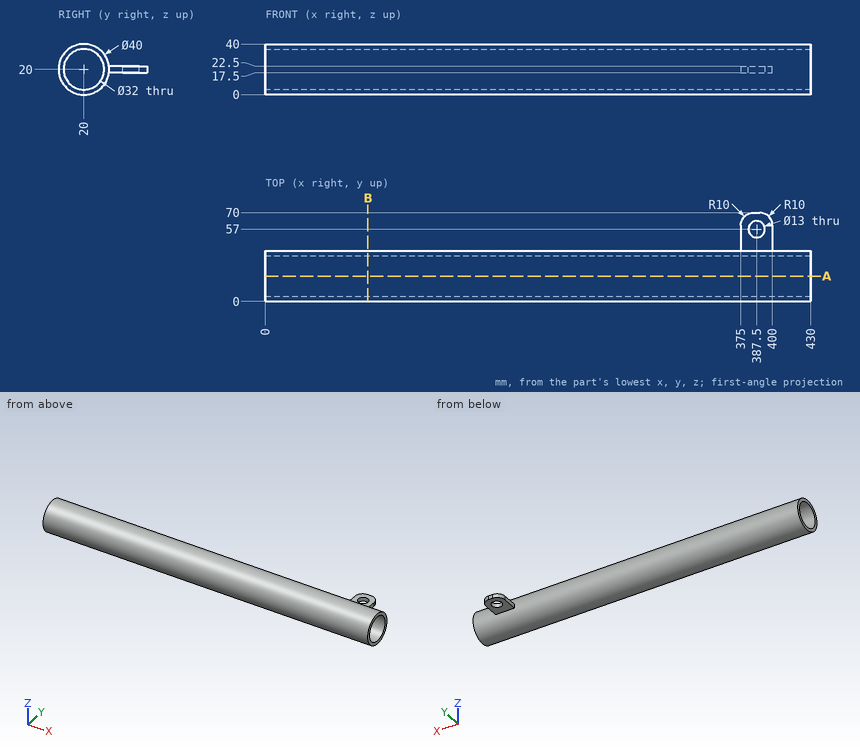
Input: dimensioned drawing with shaded views. Units: mm. Origin: part minimum x, y, z. Give positions to 0.01 mm unless a question says otherwise; leave off trailing zeros. Order: outer loops, then holes, each group sorted by start corner. A loop starts at its lowest first (then second) coordinate and runs counter-clockwise, first axis right, second up. Notation, with made-up numbers: (65.25, 35) -> (108.25, 35) arc R36 ccw to (108.25, 71) -> close; hole circle Ø7 at (87, -18). An arc over 180 degrees is marked (long way). Use a Markdown table: item, result.
1) Section query B-B, the plane x = 81. Return the cut outline in (y, z).
Answer list:
| item | result |
|---|---|
| outline | circle Ø40 at (20, 20); hole circle Ø32 at (20, 20) |
2) Ray query, line 1 along Y through (x, z) = (387.5, 20.2); line 2 along Y through (x, z) = (48, 18.5); line 3 along Y through (x, z) = (158, 20). Return the intervals inside material, ascending. Write a range as [from, to].
Answer list:
| item | result |
|---|---|
| line 1 | [0, 4], [36, 50.5], [63.5, 70] |
| line 2 | [0.06, 4.07], [35.93, 39.94] |
| line 3 | [0, 4], [36, 40] |
3) Contact query for flat-ended pins moving along their axis: P1, Ø2, axis at x = 340.5, z = 8.5, coming from the +Y side; P2, Ø1.5, axis at y = 52, z = 19, coming from the -X side; P3, Ø17, axis at x = 387.5, y = 57, coming from the +Z side. Output: stop coordinate, or through.
Answer list:
| item | result |
|---|---|
| P1 | y = 37.02 |
| P2 | x = 375 |
| P3 | z = 22.5 |
4) Section query A-A, the plane y = 20. Return the cut outline in (x, z).
Answer list:
| item | result |
|---|---|
| outline | (0, 0) -> (430, 0) -> (430, 4) -> (0, 4) -> close; (0, 36) -> (430, 36) -> (430, 40) -> (0, 40) -> close |
